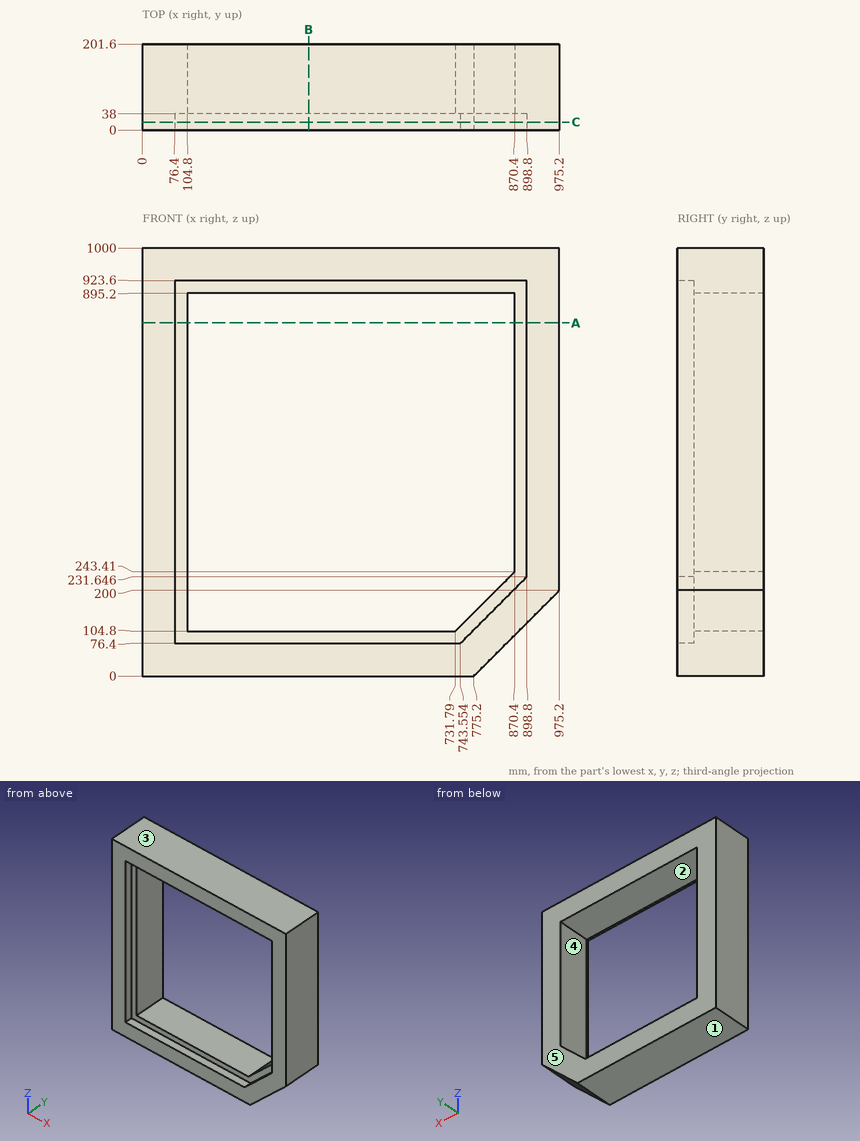
Study the drawing (mm; zero at the part's minimum x, y, z) and answer. A direction names the side the tool comes from. Give positions to 0.01 mm unless a question says otherwise; leave off trailing zeros. Loops run counter-clockwise (first coordinate to the right, second up) from the corner with the lowest first, then second, coordinate; pieces in that order, holes last. Notation, with made-up numbers: (8.25, 70) - (58.25, 70) arc R22 cw to (58.25, 87) - close; hole circle Ø4 at (73.25, 73.25). An arc over 180 degrees is marked (long way). Return JSON: item names as keys, results as strings. Group by question number.
1. Given pin 1 Ø10 at (y, z) = (175, 474) entering from -X; pin 2 Ø2 at (y, z) = (43, 107.5) entering from +X, each flat-ended and moving along its own axis, determine where each tip first touches the part or whether it passes through.
2. Determine the mould class of the marked faces 3, 4 and 5 for opening direction Z: pulls with the +Z half, pulls with the -Z half, needs draft (parallel to the pull), parting line crosses it, or undercut.
3. Find section A-A (z = 825.5). Write down the section's boundary in (x, y).
4. Find section B-B (x = 389). Write down the section's boundary in (y, z), then the cut area to 3 significant figures.
5. Find section C-C (y = 19). Write down the section's boundary in (x, z), then the cut area to 3 significant figures.
6. Which of the six approach directions +Z, -Z, +X, -X, +Y, -Y give full straight-line access (tool end or side, diameter ignored) to the marked faces 1 and 2?
7. Straight lines are drawn through the part: line 1 (Z direction, x = 115, y = 61); line 2 (X direction, y = 97, z = 316); line 3 (X direction, y = 24.5, z = 524). For each, find the intervals that lie inside material, in ascending order. Write a range as [from, to].
Verdict:
{
 "1": {"pin 1": "stops at x = 0", "pin 2": "stops at x = 883.7"},
 "2": {"face 3": "pulls with the +Z half", "face 4": "undercut", "face 5": "needs draft"},
 "3": {"outline": "(0, 0) - (76.4, 0) - (76.4, 38) - (104.8, 38) - (104.8, 201.6) - (0, 201.6) - close; (870.4, 38) - (898.8, 38) - (898.8, 0) - (975.2, 0) - (975.2, 201.6) - (870.4, 201.6) - close"},
 "4": {"outline": "(0, 0) - (201.6, 0) - (201.6, 104.8) - (38, 104.8) - (38, 76.4) - (0, 76.4) - close; (0, 923.6) - (38, 923.6) - (38, 895.2) - (201.6, 895.2) - (201.6, 1000) - (0, 1000) - close", "area": "40,100 mm^2"},
 "5": {"outline": "(0, 0) - (775.2, 0) - (975.2, 200) - (975.2, 1000) - (0, 1000) - close; hole (76.4, 76.4) - (743.55, 76.4) - (898.8, 231.65) - (898.8, 923.6) - (76.4, 923.6) - close", "area": "271,000 mm^2"},
 "6": {"face 1": "-Z, +X, -X, +Y, -Y", "face 2": "+Y, -Y"},
 "7": {"line 1": "z = [0, 104.8], [895.2, 1000]", "line 2": "x = [0, 104.8], [870.4, 975.2]", "line 3": "x = [0, 76.4], [898.8, 975.2]"}
}
